CAD build for the part. Positions are in the model's coordinates, mm. Round coordinates to 2 decimals unless told otherwise and drop trailing zeros. Loops run counter-clockwise (first coordinate to the right, second up) from the corner with the lowest first, then second, coordinate; pieces in that order, holes last. Notation, with made-up numbers: (7, 9) -> (15, 9) arc R32 cw to (15, 40) -> close; hole circle Ø5 at (35.5, 45.5). An arc over 180 degrees is marked (long way). Answer as CSV lines item,"result".
```python
from build123d import *

# Parameters (mm, degrees)
CROQUIS1_W              = 50
CROQUIS1_H              = 15
SALIENTE_EXTRUIR1_DEPTH = 15


with BuildPart() as part:
    # Croquis1 → Saliente-Extruir1 (new body)
    with BuildSketch(Plane.XY):
        Polygon((273.330497115, 777.5), (-152.038845869, -810), (-282.038845869, -810), (-273.330497115, -777.5), (152.038845869, 810), (282.038845869, 810), align=None)
        Rectangle(CROQUIS1_W, CROQUIS1_H, mode=Mode.SUBTRACT)
        with Locations((-193.593291531, -722.5)):
            Rectangle(CROQUIS1_W, CROQUIS1_H, mode=Mode.SUBTRACT)
        with Locations((-96.796645766, -361.25)):
            Rectangle(CROQUIS1_W, CROQUIS1_H, mode=Mode.SUBTRACT)
        with Locations((96.796645766, 361.25)):
            Rectangle(CROQUIS1_W, CROQUIS1_H, mode=Mode.SUBTRACT)
        with Locations((193.593291531, 722.5)):
            Rectangle(CROQUIS1_W, CROQUIS1_H, mode=Mode.SUBTRACT)
    extrude(amount=SALIENTE_EXTRUIR1_DEPTH)


solid = part.part
```
Q1. Drop flat-ended pins along their axis: pin 1 Ø7.5 at (y, z) = (-1.5, 5.5) entering from +X; pin 2 Ø4.5 at (y, z) = (-357.5, 6) entering from -X; pin 3 Ø7.5 at (y, z) = (-358, 11) entering from +X. Give the stop position or say it passes through.
Results:
pin 1,"x = 65.6"
pin 2,"x = -161.39"
pin 3,"x = -29.92"
Q2. Slice it at B-B, the plane x = -94.5. Give the cut face in (y, z), and give its area (3 significant figures).
Results:
outline,"(-595.26, 0) -> (-368.75, 0) -> (-368.75, 15) -> (-595.26, 15) -> close; (-353.75, 0) -> (-110.1, 0) -> (-110.1, 15) -> (-353.75, 15) -> close"
area,"7,050 mm2"
Q3. Slice it at D-D, the plane x = -237. Give the cut face in (y, z).
Results:
outline,"(-810, 0) -> (-641.91, 0) -> (-641.91, 15) -> (-810, 15) -> close"
Q4. Probe L1, parallel to X at y = 362.5, z = 8.5; L2, parallel to X at y = 204, z = 6; L3, parallel to X at y = -16, z = 14.25. List the from-to ranges inside material, lowest first. Write a range as [from, to].
Results:
L1,"[32.13, 71.8], [121.8, 162.13]"
L2,"[-10.34, 119.66]"
L3,"[-69.29, 60.71]"
Q5. Slice it at C-C, the plane y = 697. Give the cut face in (x, z), and give its area (3 significant figures).
Results:
outline,"(121.76, 0) -> (251.76, 0) -> (251.76, 15) -> (121.76, 15) -> close"
area,"1,950 mm2"
Q6. Slice it at A-A, the plane z = 11.5. Give the cut face in (x, y).
Results:
outline,"(-282.04, -810) -> (-152.04, -810) -> (282.04, 810) -> (152.04, 810) -> close; hole (-218.59, -730) -> (-168.59, -730) -> (-168.59, -715) -> (-218.59, -715) -> close; hole (-121.8, -368.75) -> (-71.8, -368.75) -> (-71.8, -353.75) -> (-121.8, -353.75) -> close; hole (-25, -7.5) -> (25, -7.5) -> (25, 7.5) -> (-25, 7.5) -> close; hole (71.8, 353.75) -> (121.8, 353.75) -> (121.8, 368.75) -> (71.8, 368.75) -> close; hole (168.59, 715) -> (218.59, 715) -> (218.59, 730) -> (168.59, 730) -> close"
